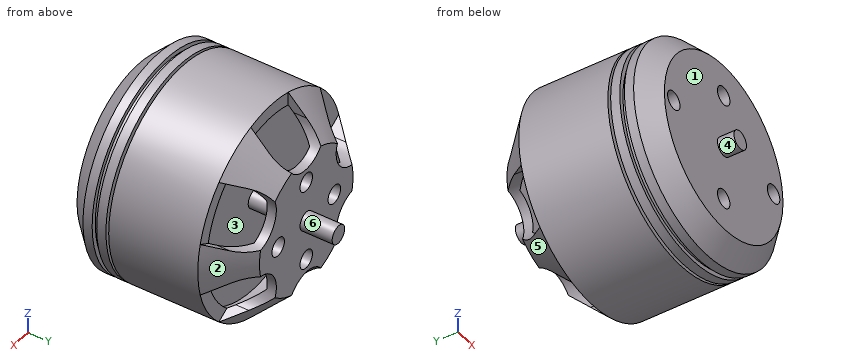
```python
from build123d import *

# Parameters (mm, degrees)
SKETCH2_R          = 1
CUT_EXTRUDE1_DEPTH = 4
SKETCH3_R          = 1
CUT_EXTRUDE2_DEPTH = 3


with BuildPart() as part:
    # Sketch1 → Revolve1 (revolve)
    with BuildSketch(Plane.XY, mode=Mode.PRIVATE) as revolve1_sk:
        Polygon((0, 18.470552147), (0, 0), (0, -5.329447853), (1, -5.329447853), (1, -3.529447853), (9.5, -3.529447853), (11.5, -1.529447853), (11.5, -0.529447853), (11, -0.529447853), (11, -0.029447853), (11.5, -0.029447853), (11.5, 0.970552147), (9.5, 0.970552147), (9.5, 1.270552147), (11.5, 1.270552147), (11.5, 10.970552147), (7.5, 14.970552147), (1, 14.970552147), (1, 18.470552147), align=None)
        Polygon((2, 13.970552147), (7.085786438, 13.970552147), (10.5, 10.556338585), (10.5, 9.331929575), (1, 9.331929575), (1, 12.970552147), (2, 12.970552147), align=None, mode=Mode.SUBTRACT)
    revolve(revolve1_sk.sketch.rotate(Axis((0, 18.470552147, 0), (0, -1, 0)), 90), axis=Axis((0, 18.470552147, 0), (0, -1, 0)))

    # Sketch2 → Cut-Extrude1 (cut)
    with BuildSketch(Plane(origin=(0, 14.970552147, 0), x_dir=(1, 0, 0), z_dir=(0, 1, 0))):
        with Locations(Location((0, -4.5, 0), (0, 0, 270))):
            Circle(SKETCH2_R)
        with Locations(Location((-4.5, 0, 0), (0, 0, 270))):
            Circle(SKETCH2_R)
        with Locations(Location((0, 4.5, 0), (0, 0, 270))):
            Circle(SKETCH2_R)
        with Locations(Location((4.5, 0, 0), (0, 0, 270))):
            Circle(SKETCH2_R)
        with BuildLine():
            Line((-3, 9), (-3, 15.381415119))
            Line((-3, 15.381415119), (3, 15.381415119))
            Line((3, 15.381415119), (3, 9))
            ThreePointArc((3, 9), (0, 6), (-3, 9))
        make_face()
        with BuildLine():
            Line((14.820696239, 5.092631348), (9.294228634, 1.901923789))
            ThreePointArc((9.294228634, 1.901923789), (5.196152423, 3), (6.294228634, 7.098076211))
            Line((6.294228634, 7.098076211), (11.820696239, 10.288783771))
            Line((11.820696239, 10.288783771), (14.820696239, 5.092631348))
        make_face()
        with BuildLine():
            Line((11.820696239, -10.288783771), (6.294228634, -7.098076211))
            ThreePointArc((6.294228634, -7.098076211), (5.196152423, -3), (9.294228634, -1.901923789))
            Line((9.294228634, -1.901923789), (14.820696239, -5.092631348))
            Line((14.820696239, -5.092631348), (11.820696239, -10.288783771))
        make_face()
        with BuildLine():
            Line((-3, -15.381415119), (-3, -9))
            ThreePointArc((-3, -9), (0, -6), (3, -9))
            Line((3, -9), (3, -15.381415119))
            Line((3, -15.381415119), (-3, -15.381415119))
        make_face()
        with BuildLine():
            Line((-14.820696239, -5.092631348), (-9.294228634, -1.901923789))
            ThreePointArc((-9.294228634, -1.901923789), (-5.196152423, -3), (-6.294228634, -7.098076211))
            Line((-6.294228634, -7.098076211), (-11.820696239, -10.288783771))
            Line((-11.820696239, -10.288783771), (-14.820696239, -5.092631348))
        make_face()
        with BuildLine():
            Line((-11.820696239, 10.288783771), (-6.294228634, 7.098076211))
            ThreePointArc((-6.294228634, 7.098076211), (-5.196152423, 3), (-9.294228634, 1.901923789))
            Line((-9.294228634, 1.901923789), (-14.820696239, 5.092631348))
            Line((-14.820696239, 5.092631348), (-11.820696239, 10.288783771))
        make_face()
    extrude(amount=-CUT_EXTRUDE1_DEPTH, mode=Mode.SUBTRACT)

    # Sketch3 → Cut-Extrude2 (cut)
    with BuildSketch(Plane.XZ.offset(3.529447853)):
        with Locations(Location((0, 6, 0), (0, 0, 270))):
            Circle(SKETCH3_R)
        with Locations(Location((0, -6, 0), (0, 0, 270))):
            Circle(SKETCH3_R)
        with Locations(Location((-8, 0, 0), (0, 0, 270))):
            Circle(SKETCH3_R)
        with Locations(Location((8, 0, 0), (0, 0, 270))):
            Circle(SKETCH3_R)
    extrude(amount=-CUT_EXTRUDE2_DEPTH, mode=Mode.SUBTRACT)


solid = part.part
```
The model under review builds one solid part; all positions refer to its coordinate system, in mm. Face numbers are marked on the shaded views. A direction names the side the tool comes from. Round coordinates to 2 decimals unless told otherwise and drop trailing zeros. Order: outer loops, then holes, each group sorted by start corner. A loop starts at its lowest first (then second) coordinate and runs counter-clockwise, first axis right, second up. Notation, with made-up numbers: (-39, -11.75) -> (-14, -11.75) arc R18 ccw to (-14, 20.25) -> close; hole circle Ø4 at (-31, 64.25). An arc over 180 degrees is marked (long way). One line per item, written item: value. Start each with the question number.
Q1. Mouldability with a two-part tool opening along Z and no side actions: class the marked faces 1, 2 and 3 as released by +Z, released by -Z, zero draft, split by the parting line, or undercut.
Q2. Take a section at A-A (y = 5.75). Write out the cut boundary in (x, z), and give its area (3 significant figures).
Q3. Machinability: for the marked faces 4, 5 and 6, which of the approach directions +Z, -Z, +X, -X, +Y, -Y give a long, thin tool a straight path to every point of the face, cutting with its end or side? Answer none if there is none.
Q4. Wall thickness on line 1 (Y direction, x = 4, z = 10.5); line 2 (X direction, y = 9.75, z = 0); line 3 (X direction, y = 14.35, z = -4.5): over which ranges is each line inside the solid? List them lowest first.
Q5. Clearance check with flat-ended pins moving along their axes: pin 1 Ø6 at (x, z) = (9, -2) entering from -Y; pin 2 Ø0.9 at (x, z) = (0.5, -11) entering from +Y; pin 3 Ø1.6 at (x, z) = (0, 4.5) entering from +Y. State where each tip first meets the part, or that it passes through.
Q6. Take a section at B-B (y = 12). Count the separate pieces of the cut face and the enclosed holes in it, and give its area (3 significant figures).
Reported:
1. face 1: zero draft
1. face 2: split by the parting line
1. face 3: undercut
2. outline: circle Ø23 at (0, 0)
2. area: 415 mm2
3. face 4: -Y
3. face 5: -Z, -X, +Y
3. face 6: +Y
4. line 1: y = -1.79 to -0.53, -0.03 to 0.97, 1.27 to 11.23
4. line 2: x = -11.5 to -10.5, -1 to 1, 10.5 to 11.5
4. line 3: x = -4.79 to -1, 1 to 4.79
5. pin 1: stops at y = -3.53
5. pin 2: stops at y = 10.97
5. pin 3: stops at y = 9.33
6. separate pieces: 7
6. enclosed holes: 0
6. area: 38.2 mm2
